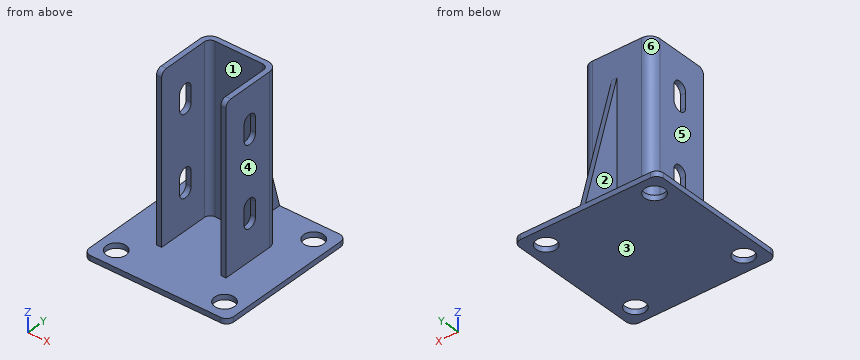
```python
from build123d import *

# Parameters (mm, degrees)
SKETCH_W     = 100
SKETCH_H     = 100
SKETCH_R     = 6.9
PAD_DEPTH    = 3.6
PAD001_DEPTH = 115
POCKET_DEPTH = 74.101
PAD002_DEPTH = 3.6
FILLET_R     = 5
FILLET001_R  = 4
FILLET002_R  = 7


with BuildPart() as part:
    # Sketch → Pad (new body)
    with BuildSketch(Plane.XY):
        Rectangle(SKETCH_W, SKETCH_H)
        with Locations((37.5, 37.5)):
            Circle(SKETCH_R, mode=Mode.SUBTRACT)
        with Locations((-37.5, 37.5)):
            Circle(SKETCH_R, mode=Mode.SUBTRACT)
        with Locations((37.5, -37.5)):
            Circle(SKETCH_R, mode=Mode.SUBTRACT)
        with Locations((-37.5, -37.5)):
            Circle(SKETCH_R, mode=Mode.SUBTRACT)
    extrude(amount=PAD_DEPTH)

    # Sketch001 (on Face10 of Pad) → Pad001 (join)
    with BuildSketch(Plane.XY.offset(3.6)):
        Polygon((-20.5, -20), (-20.5, 20), (20.5, 20), (20.5, -20), (24.1, -20), (24.1, 23.6), (-24.1, 23.6), (-24.1, -20), align=None)
    extrude(amount=PAD001_DEPTH)

    # Sketch002 (on Face15 of Pad001) → Pocket (cut, through all)
    with BuildSketch(Plane.YZ.offset(24.1)):
        with BuildLine():
            ThreePointArc((4.9, 95), (0, 99.9), (-4.9, 95))
            Line((-4.9, 95), (-4.9, 85))
            ThreePointArc((-4.9, 85), (0, 80.1), (4.9, 85))
            Line((4.9, 95), (4.9, 85))
        make_face()
        with BuildLine():
            ThreePointArc((4.9, 40), (0, 44.9), (-4.9, 40))
            Line((-4.9, 40), (-4.9, 30))
            ThreePointArc((-4.9, 30), (0, 25.1), (4.9, 30))
            Line((4.9, 40), (4.9, 30))
        make_face()
    extrude(amount=-POCKET_DEPTH, mode=Mode.SUBTRACT)

    # Sketch003 → Pad002 (join)
    with BuildSketch(Plane.YZ):
        Polygon((23.6, 100), (50, 3.6), (23.6, 3.6), align=None)
    extrude(amount=PAD002_DEPTH)

    # Fillet
    fillet_edges = [part.edges().sort_by_distance(p)[0] for p in [
        (-50, 50, 1.8),
        (-50, -50, 1.8),
        (50, -50, 1.8),
        (50, 50, 1.8),
    ]]
    fillet(fillet_edges, radius=FILLET_R)

    # Fillet001
    fillet001_edges = [part.edges().sort_by_distance(p)[0] for p in [
        (22.3, -20, 118.6),
        (-22.3, -20, 118.6),
        (20.5, 20, 61.1),
        (-20.5, 20, 61.1),
    ]]
    fillet(fillet001_edges, radius=FILLET001_R)

    # Fillet002
    fillet002_edges = [part.edges().sort_by_distance(p)[0] for p in [
        (24.1, 23.6, 61.1),
        (-24.1, 23.6, 61.1),
    ]]
    fillet(fillet002_edges, radius=FILLET002_R)


solid = part.part
```
CAD build for the part. Positions are in the model's coordinates, mm. Face numbers are marked on the shaded views. A direction names the side the tool comes from. Coordinates: 2 decimals unless noted, no trailing zeros. Write each loop counter-clockwise with the first axis right and the second up, starting at its lowest first coordinate (ties: lowest second). Pieces come first, ordered by that corner, then holes.
(1) Flat gauge pins, fed straight in: pin 1 (4 mm diameter, centred on x = 22, z = 36.5, fed in from +Y); pin 2 (6 mm diameter, centred on y = 22.5, z = 50, fed in from -X); pin 3 (3 mm diameter, centred on x = 39, y = -11.5, fed in from -Z); pin 4 (12.5 mm diameter, centred on x = -37.5, y = -37.5, fed in from -Z). Where does each tip first touch, or does it go through?
(2) Drill centre lines: probe 1 along X at (y, z) = (-37, 1); probe 2 along Y at (x, z) = (-37.5, 1.25); probe 3 along X at (y, z) = (6, 12). Where is each one in solid material? Low to high.
(3) Two-plate mould, pull along X, no slides. Class the marked faces 1, 2 and 3: +X half, -X half, draft (parallel to the pull), parting line (faces both ways), or undercut.
(4) Cut at B-B, the plane x = 37.5. List the corners of the cut face in (y, z).
(5) Cut at A-A, the plane y = 0. List the corners of the cut face in (x, z), and give its area (3 significant figures).
(6) Cut at C-C, the plane z = 98. List the corners of the cut face in (x, y), and give its area (3 significant figures).
(7) 3-axis set-ups, long thin cutter, end or side, ignore diameter. For the marked faces 4, 5 and 6: which of +Z, -Z, +X, -X, +Y, -Y reach the whole face in a straight line?
Geometry says:
1. pin 1: stops at y = 22.97
1. pin 2: stops at x = -23.47
1. pin 3: stops at z = 0
1. pin 4: passes through
2. probe 1: x = -50 to -44.38, -30.62 to 30.62, 44.38 to 50
2. probe 2: y = -50 to -44.4, -30.6 to 30.6, 44.4 to 50
2. probe 3: x = -24.1 to -20.5, 20.5 to 24.1
3. face 1: undercut
3. face 2: -X half
3. face 3: draft
4. outline: (-50, 0) - (-44.4, 0) - (-44.4, 3.6) - (-50, 3.6) - close; (-30.6, 0) - (30.6, 0) - (30.6, 3.6) - (-30.6, 3.6) - close; (44.4, 0) - (50, 0) - (50, 3.6) - (44.4, 3.6) - close
5. outline: (-50, 0) - (50, 0) - (50, 3.6) - (24.1, 3.6) - (24.1, 25.1) - (20.5, 25.1) - (20.5, 3.6) - (-20.5, 3.6) - (-20.5, 25.1) - (-24.1, 25.1) - (-24.1, 3.6) - (-50, 3.6) - close; (-24.1, 44.9) - (-20.5, 44.9) - (-20.5, 80.1) - (-24.1, 80.1) - close; (-24.1, 99.9) - (-20.5, 99.9) - (-20.5, 118.6) - (-24.1, 118.6) - close; (20.5, 44.9) - (24.1, 44.9) - (24.1, 80.1) - (20.5, 80.1) - close; (20.5, 99.9) - (24.1, 99.9) - (24.1, 118.6) - (20.5, 118.6) - close
5. area: 903 mm2
6. outline: (-24.1, -20) - (-20.5, -20) - (-20.5, -3.87) - (-24.1, -3.87) - close; (-24.1, 3.87) - (-20.5, 3.87) - (-20.5, 16) arc R4 cw to (-16.5, 20) - (16.5, 20) arc R4 cw to (20.5, 16) - (20.5, 3.87) - (24.1, 3.87) - (24.1, 16.6) arc R7 ccw to (17.1, 23.6) - (3.6, 23.6) - (3.6, 24.15) - (0, 24.15) - (0, 23.6) - (-17.1, 23.6) arc R7 ccw to (-24.1, 16.6) - close; (20.5, -20) - (24.1, -20) - (24.1, -3.87) - (20.5, -3.87) - close
6. area: 394 mm2
7. face 4: +Z, +X, +Y, -Y
7. face 5: +Z, -X, +Y, -Y
7. face 6: +Z, -X, +Y
